Drawing for the job (mm, zero at the part's lowest x, y, z). A direction names the side the tool comes from. Round coordinates to 2 decimals unless told otherwise and drop trailing zeros. Write each loop counter-clockwise with the first axis right and the second up, starting at its lowest first coordinate (ties: lowest second). Pieces come first, ordered by that corner, then holes. Notation, with made-up numbers: M 0,-13 L 51,-13 A27 cw 51,13 Z; hole C -26.5,1.5 d8. An arc over 180 degrees is marked long. Use a Markdown table: item, result. Add a question column.
1) Wall check: probe 1 along Y at (x, z) = (265, 332.5) (3 decimals); probe 2 along Z at (x, y) = (153, 122.5); probe 3 along Y at (x, z) = (395, 52). Give the ranges that are in metal, low to high.
2) Slice it at A-A on x = 450. Write the cut outline in (y, z) (3 decimals).
3) Which spindle directions (+Z, -Z, +X, -X, +Y, -Y) get a long thin tool onto all of the face, cutting with end or side? Do the marked faces 1, 2 and 3. Say none if no direction does.
4) Slice it at C-C on y = 249. Write the cut outline in (x, z), plus the area to 3 significant figures.
5) Drop a flat-ended pin along its axis: P1, Ø3, axis at x = 376, y = 170, coming from the +Z side. Give the stop position or say it passes through.
6) Slice it at B-B on z = 44. Write the cut outline in (x, y).
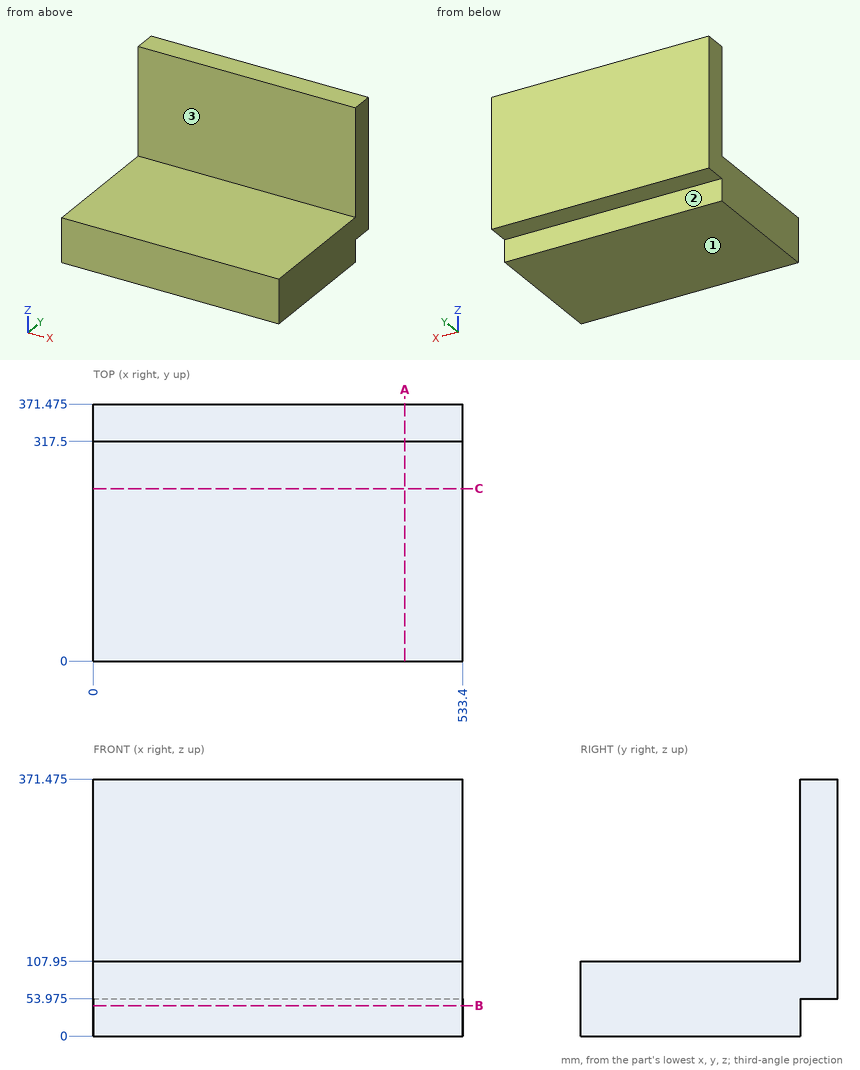
Entries:
| question | item | result |
|---|---|---|
| 1 | probe 1 | y = 317.5 to 371.475 |
| 1 | probe 2 | z = 0 to 107.95 |
| 1 | probe 3 | y = 0 to 317.5 |
| 2 | outline | M 0,0 L 317.5,0 L 317.5,53.975 L 371.475,53.975 L 371.475,371.475 L 317.5,371.475 L 317.5,107.95 L 0,107.95 Z |
| 3 | face 1 | -Z, +X, -X, +Y, -Y |
| 3 | face 2 | -Z, +X, -X, +Y |
| 3 | face 3 | +Z, +X, -X, -Y |
| 4 | outline | M 0,0 L 533.4,0 L 533.4,107.95 L 0,107.95 Z |
| 4 | area | 57,600 mm^2 |
| 5 | P1 | stops at z = 107.95 |
| 6 | outline | M 0,0 L 533.4,0 L 533.4,317.5 L 0,317.5 Z |
